Geometry: final body of the model. Coordinates: model frame, mm. Face numbers are marked on the shaded views. A direction names the side the tool comes from. Give positions to 0.01 mm unless a question says otherwise; leave off trailing zeros. Write each loop counter-clockwise with the first axis right and the second up, starting at its lowest first coordinate (ties: lowest second). Pieces come first, ordered by that corner, then holes. Notation, with made-up numbers: (71, -20) - (85, -20) arc R33 cw to (85, 10) - close; hole circle Ø3 at (14, 22.5). An arc over 180 degrees is marked (long way). Return JSON: item names as keys, results as strings.
from build123d import *

# Parameters (mm, degrees)
SKETCH1_W           = 112.8
SKETCH1_H           = 82.8
BOSS_EXTRUDE2_DEPTH = 36
SHELL1_T            = -1
SKETCH2_W           = 110.8
SKETCH2_H           = 80.8
SKETCH2_W_2         = 106.8
SKETCH2_H_2         = 76.8
BOSS_EXTRUDE3_DEPTH = 4
CUT_EXTRUDE1_REACH  = 114.8
SKETCH3_W           = 40
SKETCH3_H           = 13
BOSS_EXTRUDE4_DEPTH = 40
CUT_EXTRUDE2_REACH  = 6.2
CUT_EXTRUDE3_REACH  = 114.8
SKETCH7_R           = 2


with BuildPart() as part:
    # Sketch1 → Boss-Extrude2 (new body)
    with BuildSketch(Plane(origin=(0, 0, 0), x_dir=(1, 0, 0), z_dir=(0, 1, 0))):
        with Locations((-33.395774648, 2.631690141)):
            Rectangle(SKETCH1_W, SKETCH1_H)
    extrude(amount=BOSS_EXTRUDE2_DEPTH)

    # Shell1
    shell1_openings = [part.faces().sort_by_distance(p)[0] for p in [
        (-33.395774648, 36, -2.631690141),
    ]]
    offset(amount=SHELL1_T, openings=shell1_openings, kind=Kind.INTERSECTION)

    # Sketch2 → Boss-Extrude3 (add)
    with BuildSketch(Plane(origin=(0, 1, 0), x_dir=(1, 0, 0), z_dir=(0, 1, 0))):
        with Locations((-33.395774648, 2.631690141)):
            Rectangle(SKETCH2_W, SKETCH2_H)
        with Locations((-33.395774648, 2.631690141)):
            Rectangle(SKETCH2_W_2, SKETCH2_H_2, mode=Mode.SUBTRACT)
    extrude(amount=BOSS_EXTRUDE3_DEPTH)

    # Sketch3 → Cut-Extrude1 (cut, up to next)
    with BuildSketch(Plane(origin=(23.004225352, 0, 0), x_dir=(0, 0, -1), z_dir=(1, 0, 0)), mode=Mode.PRIVATE) as cut_extrude1_sk1:
        with Locations((2.631690141, 29.5)):
            Rectangle(SKETCH3_W, SKETCH3_H)
    cut_extrude1_tool1 = extrude(cut_extrude1_sk1.sketch, amount=-CUT_EXTRUDE1_REACH, mode=Mode.PRIVATE) & part.part
    add(cut_extrude1_tool1.solids().sort_by_distance((23.004225, 29.5, -2.63169))[0], mode=Mode.SUBTRACT)

    # Sketch4 → Boss-Extrude4 (add)
    with BuildSketch(Plane.XY.offset(-22.631690141)):
        Polygon((23.004225352, 23), (23.004225352, 16), (26.204225352, 23), align=None)
    extrude(amount=BOSS_EXTRUDE4_DEPTH)

    # Sketch6 → Cut-Extrude2 (cut, up to next)
    with BuildSketch(Plane.ZY.offset(-22.004225352), mode=Mode.PRIVATE) as cut_extrude2_sk1:
        with BuildLine():
            Line((-22.631690141, 23), (-22.560496611, 19.5))
            ThreePointArc((-22.560496611, 19.5), (-19.060496611, 16), (-15.560496611, 19.5))
            Line((-15.560496611, 19.5), (-15.560496611, 23))
            Line((-15.560496611, 23), (-22.631690141, 23))
        make_face()
    cut_extrude2_tool1 = extrude(cut_extrude2_sk1.sketch, amount=-CUT_EXTRUDE2_REACH, mode=Mode.PRIVATE) & part.part
    add(cut_extrude2_tool1.solids().sort_by_distance((22.004225, 19.832424, -19.070505))[0], mode=Mode.SUBTRACT)

    # Sketch7 → Cut-Extrude3 (cut, up to next)
    with BuildSketch(Plane(origin=(23.004225352, 0, 0), x_dir=(0, 0, -1), z_dir=(1, 0, 0)), mode=Mode.PRIVATE) as cut_extrude3_sk1:
        with Locations((36.031690141, 29)):
            Circle(SKETCH7_R)
    cut_extrude3_tool1 = extrude(cut_extrude3_sk1.sketch, amount=-CUT_EXTRUDE3_REACH, mode=Mode.PRIVATE) & part.part
    add(cut_extrude3_tool1.solids().sort_by_distance((23.004225, 29, -36.03169))[0], mode=Mode.SUBTRACT)
    # Sketch7 → Cut-Extrude3 (cut, up to next)
    with BuildSketch(Plane(origin=(23.004225352, 0, 0), x_dir=(0, 0, -1), z_dir=(1, 0, 0)), mode=Mode.PRIVATE) as cut_extrude3_sk2:
        with Locations((-30.768309859, 29)):
            Circle(SKETCH7_R)
    cut_extrude3_tool2 = extrude(cut_extrude3_sk2.sketch, amount=-CUT_EXTRUDE3_REACH, mode=Mode.PRIVATE) & part.part
    add(cut_extrude3_tool2.solids().sort_by_distance((23.004225, 29, 30.76831))[0], mode=Mode.SUBTRACT)


solid = part.part
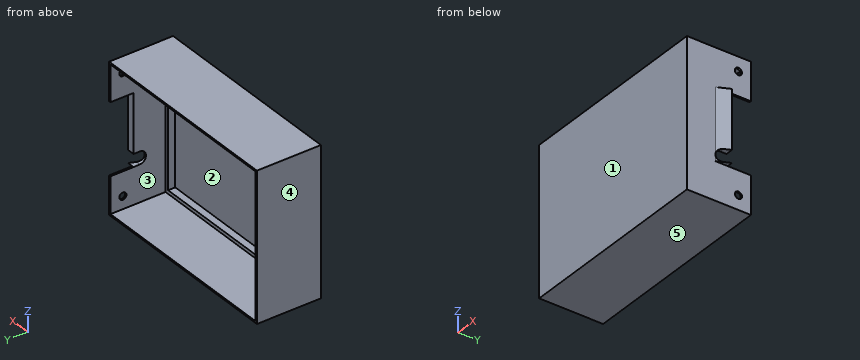
Q1. Pin query (flat end, axial travel): P1, Ø2, axis at y = 3, z = 2.5, coming from the +X side; P2, Ø1.6, axis at x = 24.5, y = 19, coming from the -Z side; P3, Ø10, axis at x = 13.5, z = 3.5, coming from the -Y side; P4, Ø1.3, axis at x = 23, z = 7, coming from the +Y side. Return the tip coordinate at first contact, or that it passes through.
Answer key:
{"P1": "stops at x = 23", "P2": "stops at z = -22.63", "P3": "stops at y = 0", "P4": "stops at y = 23"}
Q2. Section query C-C, the plane z = -7.5. Return the cut outline in (x, y), plus the area to 3 significant figures.
Answer key:
{"outline": "(-89.8, 0) - (23, 0) - (23, 16) - (26.2, 23) - (22, 23) - (22, 5) - (20, 5) - (20, 1) - (-86.8, 1) - (-86.8, 5) - (-88.8, 5) - (-88.8, 36) - (-89.8, 36) - close", "area": "197 mm^2"}
Q3. Mould query, pull axis Z, two halves, no side actions, for the marked faces 3, 4 and 5. Classes: pulls with the +Z half, pulls with the -Z half, needs draft (parallel to the pull), parting line crosses it, or undercut.
Answer key:
{"face 3": "undercut", "face 4": "needs draft", "face 5": "pulls with the -Z half"}
Q4. Section query B-B, the plane y = 29. Return the cut outline in (x, z), plus the area to 3 significant figures.
Answer key:
{"outline": "(-89.8, -44.03) - (23, -44.03) - (23, -38.03) - (22, -38.03) - (22, -43.03) - (-88.8, -43.03) - (-88.8, 37.77) - (22, 37.77) - (22, 32.77) - (23, 32.77) - (23, 38.77) - (-89.8, 38.77) - close; (22, -34.03) - (23, -34.03) - (23, -22.63) - (22, -22.63) - close; (22, 17.37) - (23, 17.37) - (23, 28.77) - (22, 28.77) - close", "area": "339 mm^2"}
Q5. Material intervals for probe 1 along Z at (x, y) = (-84, 3); probe 2 along X at (y, z) = (30.5, 20); probe 3 along Z at (x, y) = (-32, 17), sorted ascending. Write a range as [from, to].
Answer key:
{"probe 1": "z = [-44.03, -41.03], [35.77, 38.77]", "probe 2": "x = [-89.8, -88.8], [22, 23]", "probe 3": "z = [-44.03, -43.03], [37.77, 38.77]"}
Q6. Section query A-A, the plane y = 3. Return the cut outline in (x, z).
Answer key:
{"outline": "(-89.8, -44.03) - (23, -44.03) - (23, 38.77) - (-89.8, 38.77) - close; hole (-86.8, -41.03) - (20, -41.03) - (20, 35.77) - (-86.8, 35.77) - close"}
Q7. Section query D-D, the plane x = 6.5. Return the cut outline in (y, z), plus the area to 3 significant figures.
Answer key:
{"outline": "(0, -44.03) - (36, -44.03) - (36, -43.03) - (5, -43.03) - (5, -41.03) - (1, -41.03) - (1, 35.77) - (5, 35.77) - (5, 37.77) - (36, 37.77) - (36, 38.77) - (0, 38.77) - close", "area": "169 mm^2"}
Q8. Set-up query: the marked faces 1 and 2. Return all of +Z, -Z, +X, -X, +Y, -Y with unobstructed straight access to the full face (end or side cutting, diameter ignored); none if empty.
Answer key:
{"face 1": "+Z, -Z, +X, -X, -Y", "face 2": "+Y"}
